Build history of the part. All positions in model axes, mm. A direction names the side the tool comes from. Round coordinates to 2 decimals unless told otherwise and drop trailing zeros. Write each loop counter-clockwise with the first axis right and the second up, starting at its lowest first coordinate (ties: lowest second). Pieces come first, ordered by that corner, then holes. Notation, with made-up numbers: M 3.5,50 L 40.5,50 A16 cw 40.5,80 Z; hole C 53.25,75.25 d2. An arc over 180 degrees is marked long. Write item = value, one per line.
from build123d import *

# Parameters (mm, degrees)
SKETCH1_R           = 1.6500000000000001
SKETCH1_R_2         = 1.6500000000000006
BOSS_EXTRUDE1_DEPTH = 2
BOSS_EXTRUDE2_DEPTH = 2
BOSS_EXTRUDE3_DEPTH = 4
SKETCH4_R           = 1.8999999999999948
SKETCH4_R_2         = 1.8999999999999964
SKETCH4_R_3         = 1.8999999999999981
CUT_EXTRUDE1_DEPTH  = 4
SKETCH5_R           = 1.0000000000000009
SKETCH5_R_2         = 1
SKETCH5_R_3         = 1.8999999999999981
CUT_EXTRUDE2_DEPTH  = 63.418667079648536
CUT_EXTRUDE3_DEPTH  = 4
CHAMFER1_SIZE       = 5
CHAMFER2_SIZE       = 2
FILLET1_R           = 8
FILLET2_R           = 8
FILLET3_R           = 8


# Some blends are built 0.0001 mm under size
with BuildPart() as part:
    # Sketch1 → Boss-Extrude1 (new body)
    with BuildSketch(Plane.XY):
        Polygon((0, 0), (-12, -1.47e-15), (-12, 45), (0, 45), align=None)
        with Locations((-6.499999999999999, 37)):
            Circle(SKETCH1_R, mode=Mode.SUBTRACT)
        with Locations((-6.5000000000000036, 5.999999999999999)):
            Circle(SKETCH1_R_2, mode=Mode.SUBTRACT)
    extrude(amount=-BOSS_EXTRUDE1_DEPTH)

    # Sketch2 → Boss-Extrude2 (add)
    with BuildSketch(Plane(origin=(0, 0, 0), x_dir=(0, 0, -1), z_dir=(1, 0, 0))):
        Polygon((35.3, 45), (2, 0), (5.51e-15, 0), (0, 45), align=None)
    extrude(amount=BOSS_EXTRUDE2_DEPTH)

    # Sketch3 → Boss-Extrude3 (add)
    with BuildSketch(Plane(origin=(0, 45, 0), x_dir=(1, 0, 0), z_dir=(0, 1, 0))):
        Polygon((-6.1e-16, 35.3), (25, 35.3), (25.000000000000004, 1.9999999999999991), (3.47e-15, 1.9999999999999991), align=None)
    extrude(amount=-BOSS_EXTRUDE3_DEPTH)

    # Sketch4 → Cut-Extrude1 (cut)
    with BuildSketch(Plane(origin=(0, 45, 0), x_dir=(1, 0, 0), z_dir=(0, 1, 0))):
        with Locations(Location((10.199999999999998, 26.849999999999998, 0), (0, 0, 270))):
            Circle(SKETCH4_R)
        with Locations(Location((10.2, 16.45, 0), (0, 0, 270))):
            Circle(SKETCH4_R_2)
        with Locations(Location((18.999999999999996, 21.65, 0), (0, 0, 270))):
            Circle(SKETCH4_R_3)
    extrude(amount=-CUT_EXTRUDE1_DEPTH, mode=Mode.SUBTRACT)

    # Sketch5 → Cut-Extrude2 (cut, through all)
    with BuildSketch(Plane(origin=(0, 45, 0), x_dir=(1, 0, 0), z_dir=(0, 1, 0))):
        with Locations(Location((3.5826389249908894, 23.65, 0), (0, 0, 270))):
            Circle(SKETCH5_R)
        with Locations(Location((3.5826389249908894, 19.650000000000002, 0), (0, 0, 270))):
            Circle(SKETCH5_R_2)
        with Locations(Location((18.999999999999996, 21.65, 0), (0, 0, 270))):
            Circle(SKETCH5_R_3)
    extrude(amount=-CUT_EXTRUDE2_DEPTH, mode=Mode.SUBTRACT)

    # Sketch6 → Cut-Extrude3 (cut)
    with BuildSketch(Plane(origin=(0, 45, 0), x_dir=(1, 0, 0), z_dir=(0, 1, 0))):
        Polygon((10.000000000000005, 1.9999999999999991), (25.000000000000004, 16.99999999999984), (25.000000000000004, 1.9999999999999991), align=None)
    extrude(amount=-CUT_EXTRUDE3_DEPTH, mode=Mode.SUBTRACT)

    # Chamfer1
    # the kernel refuses this chamfer: 5 mm, written as the material it adds along each edge
    with BuildSketch(Plane(origin=(2, 41, -45.19841493982955), x_dir=(-0.02749587661058636, -0.9996219169112968, 0), z_dir=(0, 0, 1))) as chamfer1_piece_1_section:
        Polygon((CHAMFER1_SIZE * 0.999621916911, CHAMFER1_SIZE * 0.0274958766106), (-CHAMFER1_SIZE * 0.0274958766106, CHAMFER1_SIZE * 0.999621916911), (0, 0), align=None)
    chamfer1_piece_1 = extrude(amount=43.19841493982955, mode=Mode.PRIVATE)
    chamfer1_piece_1 = split(chamfer1_piece_1, bisect_by=Plane(origin=(3.679771833975431, 32.284665683470884, -25.89065260576845), z_dir=(0, 0.5948430054102947, 0.8038418992031009)), keep=Keep.TOP, mode=Mode.PRIVATE)
    chamfer1_piece_1 = chamfer1_piece_1 - Plane(origin=(3.5826389249908894, 39.396771086693036, -19.650000000000002), x_dir=(-1.8e-16, 0, 1), z_dir=(0, 1, 0)) * Cylinder(1, 107, mode=Mode.PRIVATE)
    chamfer1_piece_1 = chamfer1_piece_1 - Plane(origin=(3.5826389249908894, 39.396771086693036, -23.65), x_dir=(-1.8e-16, 0, 1), z_dir=(0, 1, 0)) * Cylinder(1.0000000000000009, 107, mode=Mode.PRIVATE)
    add(chamfer1_piece_1)

    # Chamfer2
    chamfer2_edges = [part.edges().sort_by_distance(p)[0] for p in [
        (1.9999999999990004, 40.50000000000074, -1.9999999999999996),
    ]]
    chamfer(chamfer2_edges, length=CHAMFER2_SIZE - 0.0001)  # a hair under: the kernel refuses the full size

    # Fillet1
    fillet1_edges = [part.edges().sort_by_distance(p)[0] for p in [
        (-12, -1.47e-15, -1),
        (-12, 45, -1),
    ]]
    fillet(fillet1_edges, radius=FILLET1_R)

    # Fillet2
    fillet2_edges = [part.edges().sort_by_distance(p)[0] for p in [
        (-6.1e-16, 43, -35.3),
        (25, 43, -35.3),
    ]]
    fillet(fillet2_edges, radius=FILLET2_R)

    # Fillet3
    fillet3_edges = [part.edges().sort_by_distance(p)[0] for p in [
        (10.000000000000005, 43, -1.9999999999999991),
        (25.000000000000004, 43, -16.99999999999984),
    ]]
    fillet(fillet3_edges, radius=FILLET3_R)


solid = part.part
1. Mould opens along X. For faces 4 (the face through (-12, 22, -1)), 5 (the face through (2.606, 40.804, -23.867)), 6 (the face through (2, 23, -8)), 7 (the face through (10.771, 43.028, -14.638)) say: pulls with the +X half, pulls with the -X half, needs draft (parallel to the pull), parting line crosses it, or undercut.
Responses:
face_4 = pulls with the -X half
face_5 = undercut
face_6 = pulls with the +X half
face_7 = undercut
2. Band-saw the part on B-B (y = 6). List the corners of the cut face in (x, z), plus the area to 3 significant figures.
Responses:
outline = M -11.75,-2 L -8.15,-2 L -8.15,0 L -11.75,0 Z; M -4.85,-2 L 0,-2 L 0,-6.44 L 2,-6.44 L 2,0 L -4.85,0 Z
area = 29.8 mm²
3. Flat gauge pins, fed straight in: pin 1 (1 mm diameter, centred on y = 12, z = -11, fed in from -X); pin 2 (10 mm diameter, centred on y = 24, z = -28.5, fed in from +X); pin 3 (5 mm diameter, centred on x = 19, z = -21.65, fed in from -Y); pin 4 (8 mm diameter, centred on y = 23.5, z = -16, fed in from +X). Where does each tip first touch, or does it go through?
Responses:
pin_1 = 0
pin_2 = through
pin_3 = 41
pin_4 = 2
4. Band-saw the part on D-D (x = -6.5). List the corners of the cut face in (y, z), plus the area to 3 significant figures.
Responses:
outline = M 0.4,-2 L 4.35,-2 L 4.35,0 L 0.4,0 Z; M 7.65,-2 L 35.35,-2 L 35.35,0 L 7.65,0 Z; M 38.65,-2 L 44.6,-2 L 44.6,0 L 38.65,0 Z
area = 75.2 mm²
5. Probe probe 1 along Y at (x, z) = (-7.5, -1); probe 2 along Y at (x, z) = (21.5, -31.5); probe 3 along Y at (x, z) = (-6.5, -1.25). List the from-to ranges inside material, lowest first.
Responses:
probe_1 = 0.81 to 4.69, 7.31 to 35.69, 38.31 to 44.19
probe_2 = 41 to 45
probe_3 = 0.4 to 4.35, 7.65 to 35.35, 38.65 to 44.6
6. Band-saw the part on C-C (z = -16.45). List the corners of the cut face in (x, y), plus the area to 3 significant figures.
Responses:
outline = M 0,19.53 L 2,19.53 L 2,36 L 7,41 L 8.3,41 L 8.3,45 L 0,45 Z; M 12.1,41 L 24.01,41 L 24.01,45 L 12.1,45 Z
area = 136 mm²
7. Tool access for faces 1 (the face through (5, 42, -2)), 2 (the face through (22.594, 42.972, -33.019)), 3 (the face through (-6, 23, -2)): list every direction of +Z, -Z, +X, -X, +Y, -Y with a clear straight run to the whole face (end or side of a thin tool).
Responses:
face_1 = +Z, +X, +Y, -Y
face_2 = -Z, +X, +Y, -Y
face_3 = -Z, -X, +Y, -Y
8. Band-saw the part on A-A (x = 19). List the corners of the cut face in (y, z), plus the area to 3 significant figures.
Responses:
outline = M 41,-35.05 L 45,-35.05 L 45,-23.55 L 41,-23.55 Z; M 41,-19.75 L 45,-19.75 L 45,-11 L 41,-11 Z
area = 81.0 mm²
